CAD build for the part. Positions are in the model's coordinates, mm. Coordinates: 2 decimals unless noted, no trailing zeros. Order: outer loops, then holes, each group sorted by start corner. A loop starts at its lowest first (then second) coordinate and runs counter-clockwise, first axis right, second up. Notation, with made-up numbers: M 89.5,67 L 116.5,67 A8 cw 116.5,72 Z; hole C 54.5,26.5 d1. An arc over 180 degrees is marked long. One line per item, written item: value.
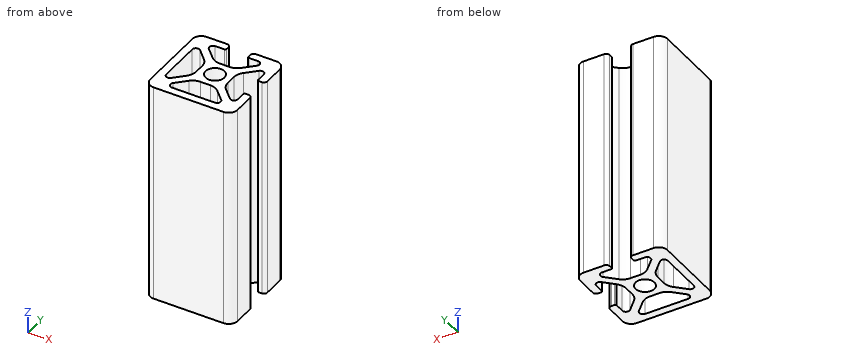
from build123d import *

# Parameters (mm, degrees)
SKETCH1_R           = 2.1463
BOSS_EXTRUDE1_DEPTH = 25.4


with BuildPart() as part:
    # Sketch1 → Boss-Extrude1 (new, symmetric)
    with BuildSketch(Plane.XY):
        with BuildLine():
            Line((-9.9949, 7.9883), (-9.9949, -7.9883))
            ThreePointArc((-9.9949, -7.9883), (-9.407180467, -9.407180467), (-7.9883, -9.9949))
            Line((-7.9883, -9.9949), (7.9883, -9.9949))
            ThreePointArc((7.9883, -9.9949), (9.407180467, -9.407180467), (9.9949, -7.9883))
            Line((9.9949, -7.9883), (9.9949, -3.2893))
            ThreePointArc((9.9949, -3.2893), (9.76427588, -2.73252412), (9.2075, -2.5019))
            Line((9.2075, -2.5019), (8.4963, -2.5019))
            ThreePointArc((8.4963, -2.5019), (8.280773853, -2.591173853), (8.1915, -2.8067))
            Line((8.1915, -2.8067), (8.1915, -4.9149))
            ThreePointArc((8.1915, -4.9149), (7.674065253, -5.689295824), (6.760603096, -5.507596904))
            Line((6.760603096, -5.507596904), (4.505765747, -3.252759555))
            ThreePointArc((4.505765747, -3.252759555), (3.856054457, -2.280397894), (3.627906192, -1.133419111))
            Line((3.627906192, -1.133419111), (3.627906192, 1.133419111))
            ThreePointArc((3.627906192, 1.133419111), (3.856054457, 2.280397894), (4.505765747, 3.252759555))
            Line((4.505765747, 3.252759555), (6.760603096, 5.507596904))
            ThreePointArc((6.760603096, 5.507596904), (7.674065253, 5.689295824), (8.1915, 4.9149))
            Line((8.1915, 4.9149), (8.1915, 2.8067))
            ThreePointArc((8.1915, 2.8067), (8.280773853, 2.591173853), (8.4963, 2.5019))
            Line((8.4963, 2.5019), (9.2075, 2.5019))
            ThreePointArc((9.2075, 2.5019), (9.76427588, 2.73252412), (9.9949, 3.2893))
            Line((9.9949, 3.2893), (9.9949, 7.9883))
            ThreePointArc((9.9949, 7.9883), (9.407180467, 9.407180467), (7.9883, 9.9949))
            Line((7.9883, 9.9949), (3.2893, 9.9949))
            ThreePointArc((3.2893, 9.9949), (2.73252412, 9.76427588), (2.5019, 9.2075))
            Line((2.5019, 9.2075), (2.5019, 8.4963))
            ThreePointArc((2.5019, 8.4963), (2.591173853, 8.280773853), (2.8067, 8.1915))
            Line((2.8067, 8.1915), (4.9149, 8.1915))
            ThreePointArc((4.9149, 8.1915), (5.689295824, 7.674065253), (5.507596904, 6.760603096))
            Line((5.507596904, 6.760603096), (3.252759555, 4.505765747))
            ThreePointArc((3.252759555, 4.505765747), (2.280397894, 3.856054457), (1.133419111, 3.627906192))
            Line((1.133419111, 3.627906192), (-1.133419111, 3.627906192))
            ThreePointArc((-1.133419111, 3.627906192), (-2.280397894, 3.856054457), (-3.252759555, 4.505765747))
            Line((-3.252759555, 4.505765747), (-5.507596904, 6.760603096))
            ThreePointArc((-5.507596904, 6.760603096), (-5.689295824, 7.674065253), (-4.9149, 8.1915))
            Line((-4.9149, 8.1915), (-2.8067, 8.1915))
            ThreePointArc((-2.8067, 8.1915), (-2.591173853, 8.280773853), (-2.5019, 8.4963))
            Line((-2.5019, 8.4963), (-2.5019, 9.2075))
            ThreePointArc((-2.5019, 9.2075), (-2.73252412, 9.76427588), (-3.2893, 9.9949))
            Line((-3.2893, 9.9949), (-7.9883, 9.9949))
            ThreePointArc((-7.9883, 9.9949), (-9.407180467, 9.407180467), (-9.9949, 7.9883))
        make_face()
        Circle(SKETCH1_R, mode=Mode.SUBTRACT)
        with BuildLine():
            Line((-6.760603096, 5.507596904), (-4.505765747, 3.252759555))
            ThreePointArc((-4.505765747, 3.252759555), (-3.856054457, 2.280397894), (-3.627906192, 1.133419111))
            Line((-3.627906192, 1.133419111), (-3.627906192, -1.133419111))
            ThreePointArc((-3.627906192, -1.133419111), (-3.856054457, -2.280397894), (-4.505765747, -3.252759555))
            Line((-4.505765747, -3.252759555), (-6.760603096, -5.507596904))
            ThreePointArc((-6.760603096, -5.507596904), (-7.674065253, -5.689295824), (-8.1915, -4.9149))
            Line((-8.1915, -4.9149), (-8.1915, 4.9149))
            ThreePointArc((-8.1915, 4.9149), (-7.674065253, 5.689295824), (-6.760603096, 5.507596904))
        make_face(mode=Mode.SUBTRACT)
        with BuildLine():
            Line((-5.507596904, -6.760603096), (-3.252759555, -4.505765747))
            ThreePointArc((-3.252759555, -4.505765747), (-2.280397894, -3.856054457), (-1.133419111, -3.627906192))
            Line((-1.133419111, -3.627906192), (1.133419111, -3.627906192))
            ThreePointArc((1.133419111, -3.627906192), (2.280397894, -3.856054457), (3.252759555, -4.505765747))
            Line((3.252759555, -4.505765747), (5.507596904, -6.760603096))
            ThreePointArc((5.507596904, -6.760603096), (5.689295824, -7.674065253), (4.9149, -8.1915))
            Line((4.9149, -8.1915), (-4.9149, -8.1915))
            ThreePointArc((-4.9149, -8.1915), (-5.689295824, -7.674065253), (-5.507596904, -6.760603096))
        make_face(mode=Mode.SUBTRACT)
    extrude(amount=BOSS_EXTRUDE1_DEPTH, both=True)


solid = part.part
Q1. Slice it at C-C (z = 8). Give the number of separate pieces and of enclosed holes in the cut face, plus the area to 3 significant figures.
Recorded:
separate pieces: 1
enclosed holes: 3
area: 201 mm^2
Q2. Slice it at A-A (y = 0). List the corners of the cut face in (x, z).
Recorded:
outline: M -9.99,-25.4 L -8.19,-25.4 L -8.19,25.4 L -9.99,25.4 Z; M -3.63,-25.4 L -2.15,-25.4 L -2.15,25.4 L -3.63,25.4 Z; M 2.15,-25.4 L 3.63,-25.4 L 3.63,25.4 L 2.15,25.4 Z
Q3. Pin check, flat tips, straight feed: pin 1 Ø1.1 at (y, z) = (0.5, 1) entering from +X; pin 2 Ø1.1 at (x, z) = (0, -7) entering from +Y; pin 3 Ø0.6 at (x, z) = (9, 0) entering from -Y. Stop position of each tip, or through.
Recorded:
pin 1: stops at x = 3.63
pin 2: stops at y = 3.63
pin 3: stops at y = -9.86
Q4. Drill centre lines: line 1 along Y through (x, z) = (0, -4.5); line 2 along X through (y, z) = (-4.5, 4). Where is each one in solid material? Low to high.
Recorded:
line 1: y = -9.99 to -8.19, -3.63 to -2.15, 2.15 to 3.63
line 2: x = -9.99 to -8.19, -5.75 to -3.25, 3.25 to 5.75, 8.19 to 9.99
